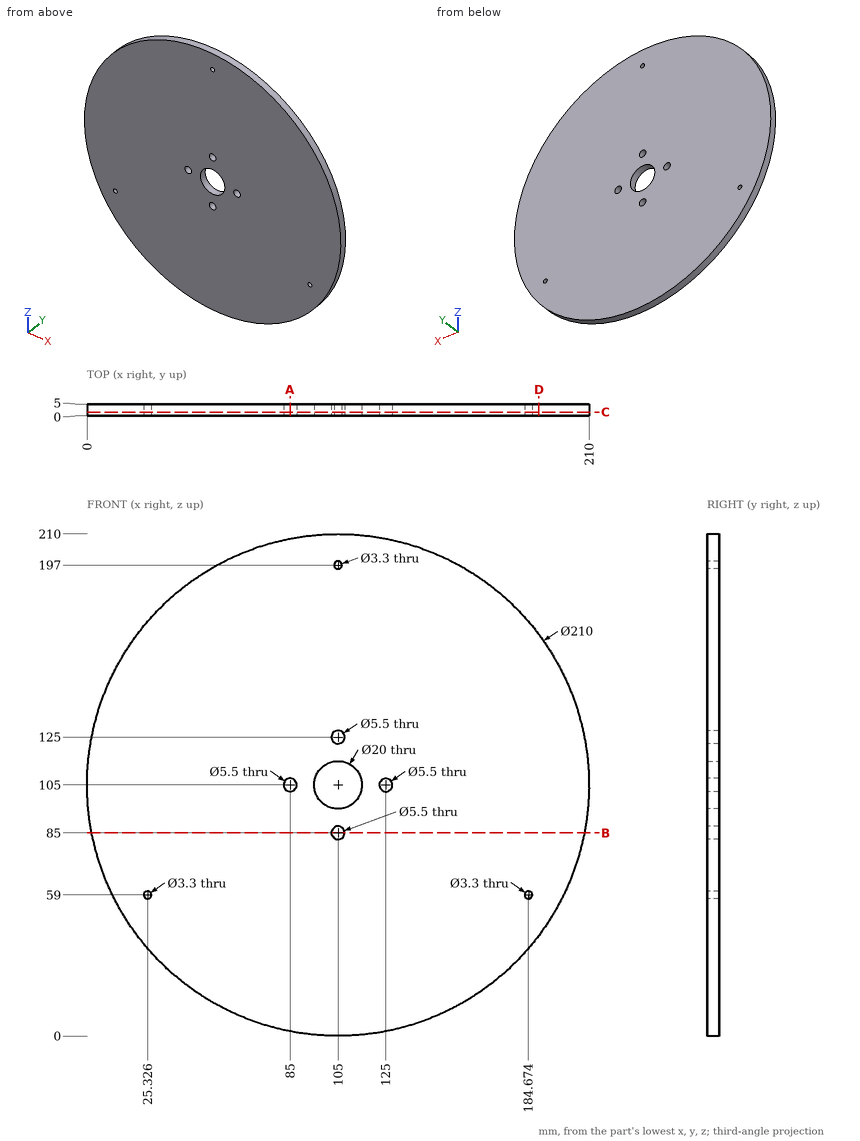
Geometry: see drawing. Coordinates: mm, zero at the bounding-box minimum. Round coordinates to 2 decimals unless told otherwise and drop trailing zeros. Loops run counter-clockwise (first coordinate to the right, second up) from the corner with the lowest first, then second, coordinate; pieces in that order, holes last. Notation, with made-up numbers: M -28,62.5 L 20,62.5 A15 ccw 20,75.5 Z; hole C 42.5,51.5 d9. An arc over 180 degrees is marked long. Use a Markdown table: item, result. Add a question column.
1. Section query B-B on z = 85. Return the cut outline in (x, y), then the cut area to 3 significant figures.
2. Section query D-D on x = 189. Return the cut outline in (y, z), then the cut area to 3 significant figures.
3. Line query: line 1 (X direction, y = 2.9, z = 105); line 2 (Z direction, x = 107, y = 3.8); line 3 (Z direction, x = 125, y = 1.8). Output: solid intervals per line, ascending.
4. Contact query for flat-ended pins moving along their axis: P1, Ø1, axis at x = 130.5, y = 2, coming from the -Z side; P2, Ø2, axis at x = 90, z = 33.5, coming from the -Y side. Output: stop coordinate, or through.
5. Section query C-C on y = 1.65. Give the number of separate pieces and of enclosed holes in the cut face, then the cut area to 3 significant figures.
6. Section query A-A on x = 85. Return the cut outline in (y, z).
Reported:
| question | item | result |
|---|---|---|
| 1 | outline | M 1.92,0 L 102.25,0 L 102.25,5 L 1.92,5 Z; M 107.75,0 L 208.08,0 L 208.08,5 L 107.75,5 Z |
| 1 | area | 1,000 mm² |
| 2 | outline | M 0,42 L 5,42 L 5,168 L 0,168 Z |
| 2 | area | 630 mm² |
| 3 | line 1 | x = 0 to 82.25, 87.75 to 95, 115 to 122.25, 127.75 to 210 |
| 3 | line 2 | z = 0.02 to 83.11, 86.89 to 95.2, 114.8 to 123.11, 126.89 to 209.98 |
| 3 | line 3 | z = 1.92 to 102.25, 107.75 to 208.08 |
| 4 | P1 | stops at z = 3.02 |
| 4 | P2 | stops at y = 0 |
| 5 | separate pieces | 1 |
| 5 | enclosed holes | 8 |
| 5 | area | 34,200 mm² |
| 6 | outline | M 0,1.92 L 5,1.92 L 5,102.25 L 0,102.25 Z; M 0,107.75 L 5,107.75 L 5,208.08 L 0,208.08 Z |
